The model under review builds one solid part; all positions refer to its coordinate system, in mm. Face numbers are marked on the shaded views. A direction names the side the tool comes from. Coordinates: 2 decimals unless noted, no trailing zeros. Write each loop counter-clockwise with the first axis right and the second up, starting at its lowest first coordinate (ties: lowest second). Pieces come first, ordered by that corner, then holes.
1) For P1, Ø1, axis at x = -5, y = 8.5, coming from the -Z side; P2, Ø6, axis at x = -0.5, y = 8, coming from the -Z side; P3, Ø8, axis at y = 2, z = 6.5, coming from the -X side (3 decimals), all flat-tipped, find the tip position at first contact; note any pin that passes through.
2) Add section A-A, the plane z = 0. State the section outline as (x, y) points, then the cut area to 3 significant figures.
3) Add section B-B, the plane x = 0. State the section outline as (y, z) points.
4) Machinability: for the marked faces 1 and 2, which of the approach directions +Z, -Z, +X, -X, +Y, -Y give a long, thin tool a straight path to every point of the face, cutting with its end or side? Answer none if there is none.
5) Add section C-C, the plane y = 9. State the section outline as (x, z) points.
6) For line 1 (X direction, y = 11, z = 0); line 2 (Y direction, x = 5.5, z = 4.25); line 3 (X direction, y = 14, z = 2), list the stretches that pass through material, from the lowest coordinate up.
7) Mouldability with a two-part tool opening along Y and no side actions: class the marked faces 3, 4, 5 and 6 as released by +Y, released by -Y, zero draft, split by the parting line, or undercut.
8) Add section D-D, the plane x = 11.4. State the section outline as (y, z) points.
from build123d import *

# Parameters (mm, degrees)
ESQUISSE2_R             = 1.6
ENL_V_MAT_EXTRU_1_DEPTH = 26.455844123
ESQUISSE3_R             = 1.65
ENL_V_MAT_EXTRU_2_DEPTH = 30.189039039


with BuildPart() as part:
    # Esquisse1 → Révolution1 (revolve)
    with BuildSketch(Plane.XY, mode=Mode.PRIVATE) as r_volution1_sk:
        Polygon((-3.03, 0), (-3.03, 16), (-6, 16), (-6, 4), (-14, 4), (-14, 0), align=None)
    revolve(r_volution1_sk.sketch.rotate(Axis((0, 0, 0), (0, 1, 0)), 270), axis=Axis((0, 0, 0), (0, 1, 0)))

    # Esquisse2 → Enlèv. mat.-Extru.1 (cut, through all)
    with BuildSketch(Plane.XZ):
        with Locations(Location((11.4, 0, 0), (0, 0, 270))):
            Circle(ESQUISSE2_R)
        with Locations(Location((-5.7, -9.872689603, 0), (0, 0, 270))):
            Circle(ESQUISSE2_R)
        with Locations(Location((-5.7, 9.872689603, 0), (0, 0, 270))):
            Circle(ESQUISSE2_R)
    extrude(amount=-ENL_V_MAT_EXTRU_1_DEPTH, mode=Mode.SUBTRACT)

    # Esquisse3 → Enlèv. mat.-Extru.2 (cut, through all)
    with BuildSketch(Plane.XY.offset(6)):
        with Locations((0, 9.5)):
            Circle(ESQUISSE3_R)
    extrude(amount=-ENL_V_MAT_EXTRU_2_DEPTH, mode=Mode.SUBTRACT)


solid = part.part
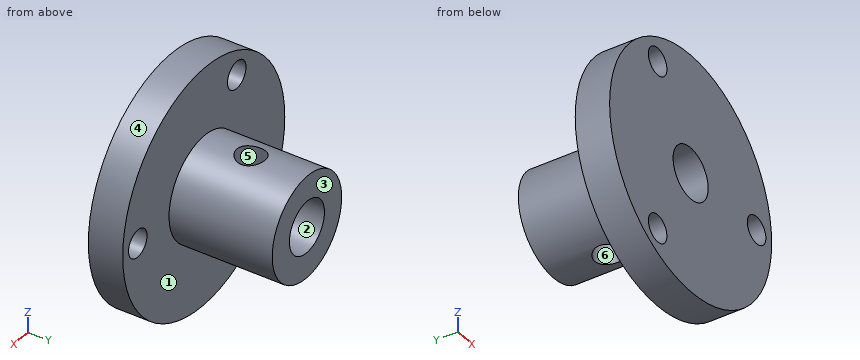
Geometry results:
1. P1: stops at z = -3.97
1. P2: stops at z = -6
1. P3: stops at x = -13.775
2. outline: (-14, 0) - (-3.03, 0) - (-3.03, 16) - (-6, 16) - (-6, 4) - (-14, 4) - close; (3.03, 0) - (9.8, 0) - (9.8, 4) - (6, 4) - (6, 16) - (3.03, 16) - close; (13, 0) - (14, 0) - (14, 4) - (13, 4) - close
2. area: 146 mm2
3. outline: (0, -14) - (4, -14) - (4, -6) - (7.85, -6) - (7.85, -3.03) - (0, -3.03) - close; (0, 3.03) - (7.85, 3.03) - (7.85, 6) - (4, 6) - (4, 14) - (0, 14) - close; (11.15, -6) - (16, -6) - (16, -3.03) - (11.15, -3.03) - close; (11.15, 3.03) - (16, 3.03) - (16, 6) - (11.15, 6) - close
4. face 1: +Y
4. face 2: +Y, -Y
5. outline: (-1.57, -5.79) - (-1.57, -2.59) arc R3.03 cw to (-1.57, 2.59) - (-1.57, 5.79) arc R6 ccw to start; (1.57, -5.79) arc R6 ccw to (1.57, 5.79) - (1.57, 2.59) arc R3.03 cw to (1.57, -2.59) - close
6. line 1: x = -6 to -3.03, 3.03 to 6
6. line 2: y = 0 to 4
6. line 3: x = -5.66 to -2.28, 2.28 to 5.66
7. face 3: released by +Y
7. face 4: zero draft
7. face 5: undercut
7. face 6: undercut
8. outline: (0, -8.13) - (4, -8.13) - (4, -1.6) - (0, -1.6) - close; (0, 1.6) - (4, 1.6) - (4, 8.13) - (0, 8.13) - close
